from build123d import *

# Parameters (mm, degrees)
SKETCH2_R            = 30
BOSS_EXTRUDE2_DEPTH  = 40.09
BOSS_EXTRUDE4_START  = 27.91
SKETCH4_R            = 30
BOSS_EXTRUDE4_DEPTH  = 27.91
SKETCH6_R            = 12.5
CUT_EXTRUDE1_DEPTH   = 19
SKETCH7_R            = 9.25
CUT_EXTRUDE2_DEPTH   = 65.815121692
CUT_EXTRUDE3_START   = -1
SKETCH8_R            = 30
SKETCH8_R_2          = 9.25
CUT_EXTRUDE3_DEPTH   = 1
CUT_EXTRUDE4_START   = -1.21
SKETCH9_R            = 30
SKETCH9_R_2          = 9.25
CUT_EXTRUDE4_DEPTH   = 1.21
SKETCH10_R           = 30
BOSS_EXTRUDE5_DEPTH  = 1
BOSS_EXTRUDE6_START  = 2
SKETCH11_R           = 9.25
BOSS_EXTRUDE6_DEPTH  = 2
SKETCH12_R           = 6.5
BOSS_EXTRUDE7_DEPTH  = 7.205952714
CUT_EXTRUDE5_START   = -5
SKETCH14_R           = 6.5
SKETCH14_R_2         = 5
CUT_EXTRUDE5_DEPTH   = 5
SKETCH15_R           = 3.25
CUT_EXTRUDE6_DEPTH   = 77.610469911
SKETCH16_R           = 30
SKETCH16_R_2         = 6.5
BOSS_EXTRUDE8_DEPTH  = 0.21
SKETCH17_R           = 30
SKETCH17_R_2         = 6.5
BOSS_EXTRUDE9_DEPTH  = 1.995952714
BOSS_EXTRUDE10_START = 0.79
SKETCH18_R           = 9.25
SKETCH18_R_2         = 3.25
BOSS_EXTRUDE10_DEPTH = 0.79
SKETCH19_R           = 9.25
SKETCH19_R_2         = 3.25
CUT_EXTRUDE7_DEPTH   = 1
BOSS_EXTRUDE11_START = 2
SKETCH21_R           = 12.5
SKETCH21_R_2         = 9.25
BOSS_EXTRUDE11_DEPTH = 2


with BuildPart() as part:
    # Sketch2 → Boss-Extrude2 (new body)
    with BuildSketch(Plane.XY):
        Circle(SKETCH2_R)
    extrude(amount=-BOSS_EXTRUDE2_DEPTH)

    # Sketch4 → Boss-Extrude4 (add)
    with BuildSketch(Plane.XY.offset(BOSS_EXTRUDE4_START)):
        Circle(SKETCH4_R)
    extrude(amount=-BOSS_EXTRUDE4_DEPTH)

    # Sketch6 → Cut-Extrude1 (cut)
    with BuildSketch(Plane.XY.offset(27.91)):
        Circle(SKETCH6_R)
    extrude(amount=-CUT_EXTRUDE1_DEPTH, mode=Mode.SUBTRACT)

    # Sketch7 → Cut-Extrude2 (cut, through all)
    with BuildSketch(Plane.XY.offset(8.91)):
        Circle(SKETCH7_R)
    extrude(amount=-CUT_EXTRUDE2_DEPTH, mode=Mode.SUBTRACT)

    # Sketch8 → Cut-Extrude3 (cut)
    with BuildSketch(Plane(origin=(0, 0, -40.09), x_dir=(-1, 0, 0), z_dir=(0, 0, -1)).offset(CUT_EXTRUDE3_START)):
        with Locations(Location((0, 0, 0), (0, 0, 180))):
            Circle(SKETCH8_R)
        with Locations(Location((0, 0, 0), (0, 0, 180))):
            Circle(SKETCH8_R_2, mode=Mode.SUBTRACT)
    extrude(amount=CUT_EXTRUDE3_DEPTH, mode=Mode.SUBTRACT)

    # Sketch9 → Cut-Extrude4 (cut)
    with BuildSketch(Plane(origin=(0, 0, -39.09), x_dir=(-1, 0, 0), z_dir=(0, 0, -1)).offset(CUT_EXTRUDE4_START)):
        with Locations(Location((0, 0, 0), (0, 0, 180))):
            Circle(SKETCH9_R)
        with Locations(Location((0, 0, 0), (0, 0, 180))):
            Circle(SKETCH9_R_2, mode=Mode.SUBTRACT)
    extrude(amount=CUT_EXTRUDE4_DEPTH, mode=Mode.SUBTRACT)

    # Sketch10 → Boss-Extrude5 (add)
    with BuildSketch(Plane(origin=(0, 0, -37.88), x_dir=(-1, 0, 0), z_dir=(0, 0, -1))):
        with Locations(Location((0, 0, 0), (0, 0, 180))):
            Circle(SKETCH10_R)
    extrude(amount=BOSS_EXTRUDE5_DEPTH)

    # Sketch11 → Boss-Extrude6 (add)
    with BuildSketch(Plane.XY.offset(-37.88).offset(BOSS_EXTRUDE6_START)):
        Circle(SKETCH11_R)
    extrude(amount=-BOSS_EXTRUDE6_DEPTH)

    # Sketch12 → Boss-Extrude7 (add)
    with BuildSketch(Plane(origin=(0, 0, -38.88), x_dir=(-1, 0, 0), z_dir=(0, 0, -1))):
        with Locations(Location((0, 0, 0), (0, 0, 180))):
            Circle(SKETCH12_R)
    extrude(amount=BOSS_EXTRUDE7_DEPTH)

    # Sketch14 → Cut-Extrude5 (cut)
    with BuildSketch(Plane(origin=(0, 0, -46.085952714), x_dir=(-1, 0, 0), z_dir=(0, 0, -1)).offset(CUT_EXTRUDE5_START)):
        Circle(SKETCH14_R)
        Circle(SKETCH14_R_2, mode=Mode.SUBTRACT)
    extrude(amount=CUT_EXTRUDE5_DEPTH, mode=Mode.SUBTRACT)

    # Sketch15 → Cut-Extrude6 (cut, through all)
    with BuildSketch(Plane.XY.offset(-35.88)):
        Circle(SKETCH15_R)
    extrude(amount=-CUT_EXTRUDE6_DEPTH, mode=Mode.SUBTRACT)

    # Sketch16 → Boss-Extrude8 (add)
    with BuildSketch(Plane(origin=(0, 0, -38.88), x_dir=(-1, 0, 0), z_dir=(0, 0, -1))):
        with Locations(Location((0, 0, 0), (0, 0, 180))):
            Circle(SKETCH16_R)
        Circle(SKETCH16_R_2, mode=Mode.SUBTRACT)
    extrude(amount=BOSS_EXTRUDE8_DEPTH)

    # Sketch17 → Boss-Extrude9 (add)
    with BuildSketch(Plane(origin=(0, 0, -39.09), x_dir=(-1, 0, 0), z_dir=(0, 0, -1))):
        with Locations(Location((0, 0, 0), (0, 0, 180))):
            Circle(SKETCH17_R)
        Circle(SKETCH17_R_2, mode=Mode.SUBTRACT)
    extrude(amount=BOSS_EXTRUDE9_DEPTH)

    # Sketch18 → Boss-Extrude10 (add)
    with BuildSketch(Plane.XY.offset(-35.88).offset(BOSS_EXTRUDE10_START)):
        Circle(SKETCH18_R)
        Circle(SKETCH18_R_2, mode=Mode.SUBTRACT)
    extrude(amount=-BOSS_EXTRUDE10_DEPTH)

    # Sketch19 → Cut-Extrude7 (cut)
    with BuildSketch(Plane.XY.offset(-35.09)):
        Circle(SKETCH19_R)
        Circle(SKETCH19_R_2, mode=Mode.SUBTRACT)
    extrude(amount=-CUT_EXTRUDE7_DEPTH, mode=Mode.SUBTRACT)

    # Sketch21 → Boss-Extrude11 (add)
    with BuildSketch(Plane.XY.offset(8.91).offset(BOSS_EXTRUDE11_START)):
        Circle(SKETCH21_R)
        Circle(SKETCH21_R_2, mode=Mode.SUBTRACT)
    extrude(amount=-BOSS_EXTRUDE11_DEPTH)


solid = part.part
Verification items for the finished model (mm, model axes). A direction names the side the tool comes from. Coordinates: 2 decimals unless noted, no trailing zeros. Order: outer loops, then holes, each group sorted by start corner. A loop starts at its lowest first (then second) coordinate and runs counter-clockwise, first axis right, second up. Notation, with made-up numbers: (24, 35) -> (54, 35) arc R25 cw to (54, 53) -> close; hole circle Ø7 at (23, 7). An arc over 180 degrees is marked (long way). Put each result on its own line as item: value. Start each with the question number.
1. Access from +Z, -Z, +X, -X, +Y, -Y to the whole of each face (thin tool, end or side, straight path). Record for faces 4 (the cylindrical face through (1.08, -4.88, -43.55)), 5 (the cylindrical face through (-2.01, -9.03, -12.26)), 6 (the flat face through (3.3, 1, -46.086)).
2. Cross-section at A-A, the plane x = 0. Record the boundary of the cut face in (y, z), then the cut area to 3 significant figures.
3. Go/stop test with flat-tipped pins: pin 1 Ø2 at (x, z) = (20, -35.5) entering from +Y; pin 2 Ø8 at (y, z) = (6, 19.5) entering from -X; pin 3 Ø2 at (x, y) = (-10.5, -16) entering from -Z; pin 4 Ø1.5 at (x, y) = (-1, 1.5) entering from +Z. Record where each tip stops, or that it passes through.
4. Cross-section at D-D, the plane y = 19.5. Record the boundary of the cut face in (x, z), then the cut area to 3 significant figures.
5. Material ranges on L1, parallel to Y at x = 0, z = -43; L2, parallel to Y at x = 0, z = -38.75; L3, parallel to Z at x = -20, y = -9, recorded low to high. Write a range as [from, to].
6. Mould release check, pull along X, two halves, no side actions. Record for faces 1 (the flat face through (13, 0, 27.91)), 2 (the cylindrical face through (-2.579, -1.978, -41.018)), 3 (the cylindrical face through (16.128, -25.296, -6.105)): released by +X, released by -X, zero draft, split by the parting line, or undercut.
7. Cross-section at C-C, the plane z = -27. Record the boundary of the cut face in (x, y).
Computed:
1. face 4: -Z
1. face 5: +Z
1. face 6: -Z, +X, -X, +Y, -Y
2. outline: (-30, -41.09) -> (-5, -41.09) -> (-5, -46.09) -> (-3.25, -46.09) -> (-3.25, -36.09) -> (-9.25, -36.09) -> (-9.25, 10.91) -> (-12.5, 10.91) -> (-12.5, 27.91) -> (-30, 27.91) -> close; (3.25, -46.09) -> (5, -46.09) -> (5, -41.09) -> (30, -41.09) -> (30, 27.91) -> (12.5, 27.91) -> (12.5, 10.91) -> (9.25, 10.91) -> (9.25, -36.09) -> (3.25, -36.09) -> close
2. area: 2,830 mm2
3. pin 1: y = 23.22
3. pin 2: x = -29.93
3. pin 3: z = -41.09
3. pin 4: through
4. outline: (-22.8, -41.09) -> (22.8, -41.09) -> (22.8, 27.91) -> (-22.8, 27.91) -> close
4. area: 3,150 mm2
5. L1: [-5, -3.25], [3.25, 5]
5. L2: [-30, -3.25], [3.25, 30]
5. L3: [-41.09, 27.91]
6. face 1: zero draft
6. face 2: undercut
6. face 3: split by the parting line
7. outline: circle Ø60 at (0, 0); hole circle Ø18.5 at (0, 0)
